Can you work these out from the model? Positions are in its coordinate system, mm. A direction names the side the tool comes from. Give positions to 0.01 mm unless a question says otherwise; leave off trailing zeros. Order: outer loops, then holes, each group sorted by start corner. A loop starts at its lowest first (then second) coordinate and runs counter-clockwise, first axis right, second up. Notation, with made-up numbers: (14, 31) - (65, 31) arc R15 cw to (65, 52) - close; hole circle Ø3 at (21, 17). An arc over 180 degrees is marked (long way). Answer as a JSON object with one key per item and string values.
```python
from build123d import *

# Parameters (mm, degrees)
SKETCH_W      = 85
SKETCH_H      = 35
SKETCH_R      = 1
PAD_DEPTH     = 2
SKETCH001_W   = 13
SKETCH001_H   = 8
SKETCH001_W_2 = 8
SKETCH001_H_2 = 21.912057
SKETCH001_W_3 = 71
SKETCH001_W_4 = 15
SKETCH001_W_5 = 23
PAD001_DEPTH  = 5


with BuildPart() as part:
    # Sketch → Pad (new body)
    with BuildSketch(Plane.YZ):
        with Locations((42.5, 17.5)):
            Rectangle(SKETCH_W, SKETCH_H)
        with Locations((2.5, 32.416278)):
            Circle(SKETCH_R, mode=Mode.SUBTRACT)
        with Locations((82.5, 32.416278)):
            Circle(SKETCH_R, mode=Mode.SUBTRACT)
        with Locations((82.5, 2.416278)):
            Circle(SKETCH_R, mode=Mode.SUBTRACT)
        with Locations((2.5, 2.416278)):
            Circle(SKETCH_R, mode=Mode.SUBTRACT)
    extrude(amount=PAD_DEPTH)

    # Sketch001 (on Face10 of Pad) → Pad001 (join)
    with BuildSketch(Plane.YZ.offset(2)):
        with Locations((73.531729, 5.652397)):
            Rectangle(SKETCH001_W, SKETCH001_H)
        with Locations((5.173597, 17.259363)):
            Rectangle(SKETCH001_W_2, SKETCH001_H_2)
        with Locations((45.234558, 29.475365)):
            Rectangle(SKETCH001_W_3, SKETCH001_H)
        with Locations((42.446848, 5.317278)):
            Rectangle(SKETCH001_W_4, SKETCH001_H)
        with Locations((21.441039, 5.114811)):
            Rectangle(SKETCH001_W_5, SKETCH001_H)
    extrude(amount=PAD001_DEPTH)


solid = part.part
```
Q1. If we section it at C-C, the plane z = 20: Please give me the cut outline in (x, y).
Recorded:
{"outline": "(0, 0) - (2, 0) - (2, 1.17) - (7, 1.17) - (7, 9.17) - (2, 9.17) - (2, 85) - (0, 85) - close"}
Q2. I need wall thicknesses on L1, parallel to Z at x = 1.55, y = 2.5; L2, parallel to Y at x = 4, z = 7.5; L3, parallel to Z at x = 5, y = 38. Which ranges of each line are inside material? Lowest first, please.
Recorded:
{"L1": "z = 0 to 1.42, 3.42 to 31.42, 33.42 to 35", "L2": "y = 1.17 to 9.17, 9.94 to 32.94, 34.95 to 49.95, 67.03 to 80.03", "L3": "z = 1.32 to 9.32, 25.48 to 33.48"}
Q3. Which directions (+Z, -Z, +X, -X, +Y, -Y) give clear straight access to the entire face, cutting with the end or side of a thin tool? Please do faces 5 (the face through (4, 34.947, 5)), 6 (the face through (4, 80.032, 6)), 7 (the face through (4, 1.174, 17)).
Recorded:
{"face 5": "-Z, +X", "face 6": "-Z, +X, +Y", "face 7": "+Z, -Z, +X, -Y"}
Q4. If we section it at B-B, the plane y = 82.5: Please give me the cut outline in (x, z), then the cut area to 3 significant figures.
Recorded:
{"outline": "(0, 0) - (2, 0) - (2, 1.42) - (0, 1.42) - close; (0, 3.42) - (2, 3.42) - (2, 31.42) - (0, 31.42) - close; (0, 33.42) - (2, 33.42) - (2, 35) - (0, 35) - close", "area": "62.0 mm^2"}
Q5. We'd pull the mould along Z, two halves only. Please class faces 1 (the face through (4, 9.174, 17)), 2 (the face through (4, 5, 28.215)), 3 (the face through (0.99, 2.28, 31.44)), 4 (the face through (4, 5, 6.303)): released by +Z, released by -Z, zero draft, split by the parting line, or undercut.
Recorded:
{"face 1": "zero draft", "face 2": "released by +Z", "face 3": "undercut", "face 4": "released by -Z"}
Q6. If we section it at A-A, the plane x = 5.75: Please give me the cut outline in (y, z), then the cut area to 3 significant figures.
Recorded:
{"outline": "(1.17, 6.3) - (9.17, 6.3) - (9.17, 28.22) - (1.17, 28.22) - close; (9.73, 25.48) - (80.73, 25.48) - (80.73, 33.48) - (9.73, 33.48) - close; (9.94, 1.11) - (32.94, 1.11) - (32.94, 9.11) - (9.94, 9.11) - close; (34.95, 1.32) - (49.95, 1.32) - (49.95, 9.32) - (34.95, 9.32) - close; (67.03, 1.65) - (80.03, 1.65) - (80.03, 9.65) - (67.03, 9.65) - close", "area": "1,150 mm^2"}
Q7. I'm going to push flat-ended pins straight in: pin 1 Ø4 at (y, z) = (59, 27.5) entering from -X; pin 2 Ø2.5 at (x, y) = (5, 71) entering from +Z; pin 3 Ø12 at (y, z) = (47.5, 16.5) entering from +X; pin 4 Ø4 at (x, z) = (5.5, 4) entering from +Y. Where does each tip first touch, or does it pass through?
Recorded:
{"pin 1": "stops at x = 0", "pin 2": "stops at z = 33.48", "pin 3": "stops at x = 2", "pin 4": "stops at y = 80.03"}
Q8. If we section it at D-D, the plane y = 14: Please give me the cut outline in (x, z), then the cut area to 3 significant figures.
Recorded:
{"outline": "(0, 0) - (2, 0) - (2, 1.11) - (7, 1.11) - (7, 9.11) - (2, 9.11) - (2, 25.48) - (7, 25.48) - (7, 33.48) - (2, 33.48) - (2, 35) - (0, 35) - close", "area": "150 mm^2"}
